Can you work these out from the model? Positions are in its coordinate system, mm. Give positions to 0.01 mm unless a question says otherwise; leave off trailing zeros. Write each loop counter-clockwise with the first axis right and the second up, starting at its lowest first coordinate (ties: lowest second). Pieces come first, ordered by that corner, then holes.
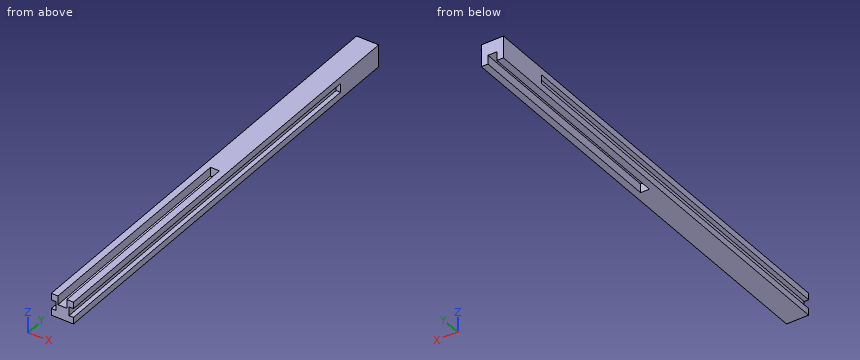
```python
from build123d import *

# Parameters (mm, degrees)
SKETCH1_W           = 10
SKETCH1_H           = 10
BOSS_EXTRUDE1_DEPTH = 200
SKETCH3_W           = 4
SKETCH3_H           = 100
CUT_EXTRUDE3_DEPTH  = 4
SKETCH5_W           = 4
SKETCH5_H           = 175
CUT_EXTRUDE4_DEPTH  = 2
SKETCH2_W           = 4
SKETCH2_H           = 100
CUT_EXTRUDE5_DEPTH  = 4
SKETCH4_W           = 4
SKETCH4_H           = 175
CUT_EXTRUDE6_DEPTH  = 2


with BuildPart() as part:
    # Sketch1 → Boss-Extrude1 (new body)
    with BuildSketch(Plane(origin=(0, 0, 0), x_dir=(1, 0, 0), z_dir=(0, 1, 0))):
        with Locations((-38.49189023, 27.694440025)):
            Rectangle(SKETCH1_W, SKETCH1_H)
    extrude(amount=BOSS_EXTRUDE1_DEPTH)

    # Sketch3 → Cut-Extrude3 (cut)
    with BuildSketch(Plane(origin=(0, 0, -32.694440025), x_dir=(-1, 0, 0), z_dir=(0, 0, -1))):
        with Locations((38.49189023, 150)):
            Rectangle(SKETCH3_W, SKETCH3_H)
    extrude(amount=-CUT_EXTRUDE3_DEPTH, mode=Mode.SUBTRACT)

    # Sketch5 → Cut-Extrude4 (cut)
    with BuildSketch(Plane.ZY.offset(43.49189023)):
        with Locations((-27.694440025, 87.5)):
            Rectangle(SKETCH5_W, SKETCH5_H)
    extrude(amount=-CUT_EXTRUDE4_DEPTH, mode=Mode.SUBTRACT)

    # Sketch2 → Cut-Extrude5 (cut)
    with BuildSketch(Plane.XY.offset(-22.694440025)):
        with Locations((-38.49189023, 50)):
            Rectangle(SKETCH2_W, SKETCH2_H)
    extrude(amount=-CUT_EXTRUDE5_DEPTH, mode=Mode.SUBTRACT)

    # Sketch4 → Cut-Extrude6 (cut)
    with BuildSketch(Plane(origin=(-33.49189023, 0, 0), x_dir=(0, 0, -1), z_dir=(1, 0, 0))):
        with Locations((27.694440025, 87.5)):
            Rectangle(SKETCH4_W, SKETCH4_H)
    extrude(amount=-CUT_EXTRUDE6_DEPTH, mode=Mode.SUBTRACT)


solid = part.part
```
1) For pin 1 Ø1.6 at (x, z) = (-34.5, -28) entering from -Y; pin 2 Ø1.2 at (x, y) = (-39.5, 144.5) entering from -Z; pin 3 Ø2 at (x, y) = (-38.5, 32.5) entering from +Z, each with a flat end and sliding along its axis, tell me the tip position at first contact or that it passes through.
Values follow:
pin 1: stops at y = 175
pin 2: stops at z = -28.69
pin 3: stops at z = -26.69
2) Suppose I cut it at A-A on x = -38. Write out the boundary of the cut face in (y, z).
Values follow:
outline: (0, -32.69) - (100, -32.69) - (100, -28.69) - (200, -28.69) - (200, -22.69) - (100, -22.69) - (100, -26.69) - (0, -26.69) - close
3) Please list where these lines run through material, in increasing order: L1, parallel to X at y = 85.5, z = -24.25; L2, parallel to Z at x = -33.75, y = 27; L3, parallel to X at y = 18, z = -26.5.
Values follow:
L1: x = -43.49 to -40.49, -36.49 to -33.49
L2: z = -32.69 to -29.69, -25.69 to -22.69
L3: x = -41.49 to -40.49, -36.49 to -35.49
4) Suppose I cut it at B-B on y = 14.5. Write out the boundary of the cut face in (x, z).
Values follow:
outline: (-43.49, -32.69) - (-33.49, -32.69) - (-33.49, -29.69) - (-35.49, -29.69) - (-35.49, -25.69) - (-33.49, -25.69) - (-33.49, -22.69) - (-36.49, -22.69) - (-36.49, -26.69) - (-40.49, -26.69) - (-40.49, -22.69) - (-43.49, -22.69) - (-43.49, -25.69) - (-41.49, -25.69) - (-41.49, -29.69) - (-43.49, -29.69) - close
